The figure shows three views and two pictorial views of one solid part (mm, origin at its lowest corner). Answer the questions. A direction names the side the tool comes from. Coordinates: 2 decimals unless noted, no trailing zeros. Loops run counter-clockwise (first coordinate to the right, second up) from the corner with the lowest first, then second, coordinate; pieces in that order, holes last. Notation, with made-up numbers: M -12.5,-17.5 L 34.5,-17.5 A33 ccw 34.5,20.5 Z; hole C -28.5,27.5 d7. An arc over 180 degrees is marked long. Write each question's results on one line, items separated by ' | '.
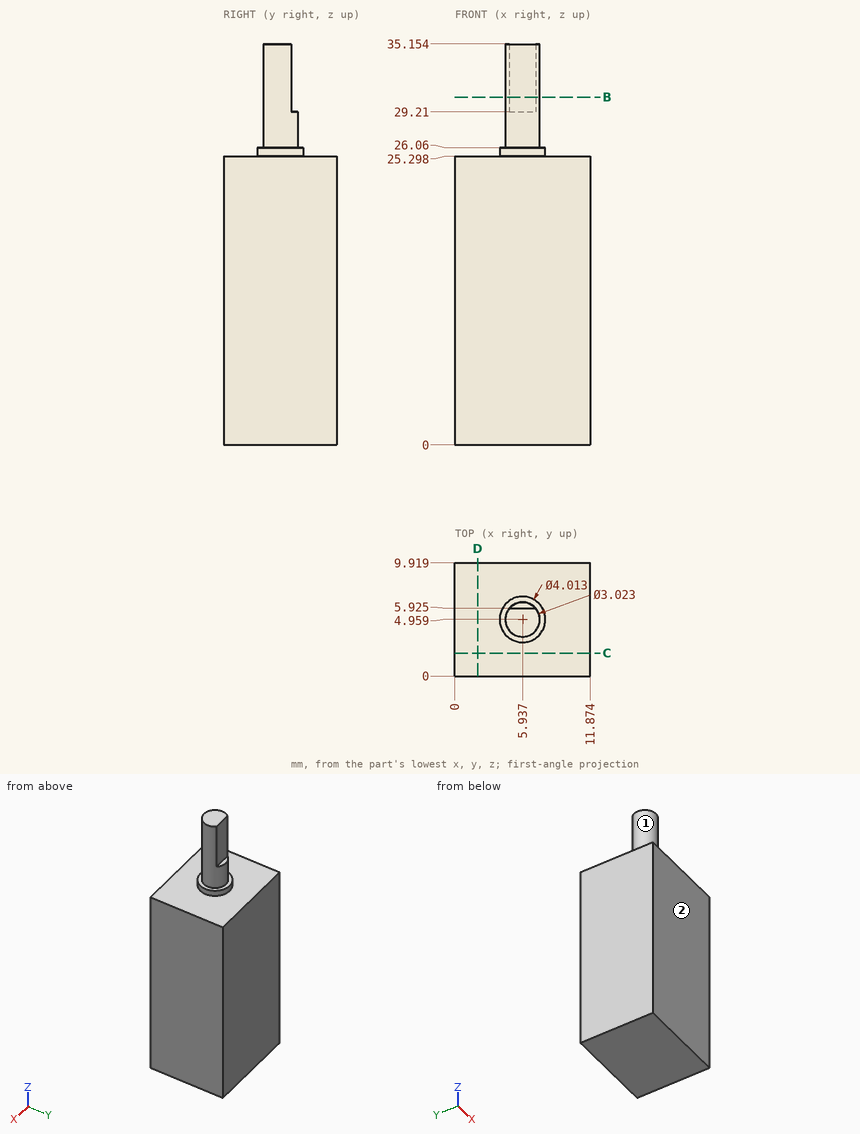
1) Find section B-B, the plane z = 30.5. Give the vertices of the cut face in (x, y) (1 decimal).
Check result:
outline: M 4.8,5.9 A1.5 ccw long 7.1,5.9 Z
2) Given pin 1 Ø3 at (y, z) = (7.5, 30.5) entering from +X; pin 2 Ø1.2 at (x, z) = (6.5, 32.5) entering from +Y (1 decimal), each flat-ended and moving along its own axis, determine where each tip first touches the part or whether it passes through.
Check result:
pin 1: through | pin 2: y = 5.9
3) Find section D-D, the plane x = 2. Give the vertices of the cut face in (y, z).
Check result:
outline: M 0,0 L 9.92,0 L 9.92,25.3 L 0,25.3 Z
4) Which of the six approach directions +Z, -Z, +X, -X, +Y, -Y give full straight-line access (tool end or side, diameter ignored) to the marked faces 1 and 2?
Check result:
face 1: +Z | face 2: +Z, -Z, +X, -X, -Y
5) Find section C-C, the plane y = 2. Give the vertices of the cut face in (x, z) (1 decimal), and give its area (3 significant figures).
Check result:
outline: M 0,0 L 11.9,0 L 11.9,25.3 L 0,25.3 Z | area: 300 mm^2
6) A straight line is drawn through the part: probe 1 along Z at (x, y) = (10.5, 8.25). Find the intervals that lie inside material, in ascending order. Write a range as [from, to].
Check result:
probe 1: [0, 25.3]
